Geometry: final body of the model. Coordinates: model frame, mm. A direction names the side the tool comes from. Coordinates: 2 decimals unless noted, no trailing zeros. Write each loop counter-clockwise with the first axis right and the second up, starting at its lowest first coordinate (ties: lowest second). Pieces come first, ordered by that corner, then holes. Notation, with made-up numbers: (49, 13) -> (97, 13) arc R17 cw to (97, 31) -> close; hole circle Ø10 at (8.25, 7.5). An arc over 180 degrees is marked (long way). Answer as a JSON object with one key per item and string values. Group by question number.
```python
from build123d import *

# Parameters (mm, degrees)
F1_DEPTH = 6
F3_DEPTH = 2
F4_R     = 2.25
F5_DEPTH = 8.001
F6_R     = 3.75
F7_DEPTH = 2
F8_SIZE  = 3


with BuildPart() as f1:
    # F0 (on Top) → F1 (new body)
    with BuildSketch(Plane.XY):
        Polygon((-30, 0), (-10, 0), (-10, -40), (0, -40), (10, -40), (10, 0), (30, 0), (30, 20), (0, 20), (-30, 20), align=None)
    extrude(amount=F1_DEPTH)

    # F2 (on face) → F3 (join)
    with BuildSketch(Plane.XY.offset(6)):
        Polygon((2.71, 0), (0, 0), (-2.71, 0), (-2.71, -40), (2.71, -40), align=None)
        Polygon((30, 7.29), (30, 12.71), (-30, 12.71), (-30, 10), (-30, 7.29), align=None)
    extrude(amount=F3_DEPTH)

    # F4 (on face) → F5 (cut, through all)
    with BuildSketch(Plane(origin=(0, 0, 0), x_dir=(1, 0, 0), z_dir=(0, 0, -1))):
        with Locations((-20, -10)):
            Circle(F4_R)
        with Locations((0, 10)):
            Circle(F4_R)
        with Locations((0, 30)):
            Circle(F4_R)
        with Locations((20.741304, -10)):
            Circle(F4_R)
        with Locations((0, -10)):
            Circle(F4_R)
    extrude(amount=-F5_DEPTH, mode=Mode.SUBTRACT)

    # F6 (on face) → F7 (cut)
    with BuildSketch(Plane(origin=(0, 0, 0), x_dir=(1, 0, 0), z_dir=(0, 0, -1))):
        with Locations((0, 30)):
            Circle(F6_R)
        with Locations((0, 10)):
            Circle(F6_R)
        with Locations((20.741304, -10)):
            Circle(F6_R)
        with Locations((-20, -10)):
            Circle(F6_R)
        with Locations((0, -10)):
            Circle(F6_R)
    extrude(amount=-F7_DEPTH, mode=Mode.SUBTRACT)

    # F8
    f8_edges = [f1.edges().sort_by_distance(p)[0] for p in [
        (-10, -20, 0),
        (-20, 0, 0),
        (10, -20, 0),
        (20, 0, 0),
        (0, 20, 0),
        (30, 10, 0),
        (-30, 10, 0),
        (0, -40, 0),
    ]]
    chamfer(f8_edges, length=F8_SIZE)


solid = f1.part
```
Item 1: Mould query, pull axis Y, two halves, no side actions, for faces 5 (the flat face through (2, -28, 2)), 6 (the flat face through (-30, 10, 5)), 7 (the flat face through (18, 1, 2)). Classes: +Y half, -Y half, draft (parallel to the pull), parting line (faces both ways), or undercut.
Item 2: Section A-A on z = 6.75. Output: boundary loops of the cut face in (x, y).
Item 3: Contact query for flat-ended pins moving along their axis: pin 1 (3.5 mm diameter, centred on x = 16.5, z = 4, fed in from -Y); pin 2 (8 mm diameter, centred on x = -21.5, y = 11, fed in from -Z); pin 3 (0.6 mm diameter, centred on y = -29.5, z = 6.5, fed in from -X); pin 4 (1.6 mm diameter, centred on x = -10.5, z = 7, fed in from -Y). Output: stop coordinate, or through.
Item 4: Set-up query: faces 1 (the cylindrical face through (-0.488, -13.718, 0.986)), 2 (the flat face through (9, -19, 2)), 3 (the flat face through (2.71, -20, 7)), 4 (the flat face through (20, 0, 4)). Return all of +Z, -Z, +X, -X, +Y, -Y with unobstructed straight access to the full face (end or side cutting, diameter ignored); none if empty.
Item 5: Section B-B on x = -20. Output: boundary loops of the cut face in (y, z), then the cut area to 3 significant figures.
Item 6: Section C-C on y = 10. Give the number of separate pieces and of enclosed holes in the cut face, then the cut area to 3 significant figures.
Item 7: Ray query, L1, parallel to X at y = 10, z = 5.75; L2, parallel to X at y = 11, z = 6; L3, parallel to Y at x = -20, z = 3.4. Return the intervals inside material, ascending. Write a range as [from, to].
Item 8: Section D-D on y = -30. Output: boundary loops of the cut face in (x, z).
Answer sheet:
{
 "1": {"face 5": "undercut", "face 6": "draft", "face 7": "-Y half"},
 "2": {"outline": "(-30, 7.29) -> (30, 7.29) -> (30, 12.71) -> (-30, 12.71) -> close; (-2.71, -40) -> (2.71, -40) -> (2.71, 0) -> (-2.71, 0) -> close; hole circle Ø4.5 at (-20, 10); hole circle Ø4.5 at (0, -30); hole circle Ø4.5 at (0, -10); hole circle Ø4.5 at (0, 10); hole circle Ø4.5 at (20.74, 10)"},
 "3": {"pin 1": "stops at y = 0", "pin 2": "stops at z = 0", "pin 3": "stops at x = -2.71", "pin 4": "stops at y = 7.29"},
 "4": {"face 1": "-Z", "face 2": "-Z, +X, -Y", "face 3": "+Z, +X, -Y", "face 4": "+Z, -Z, +X, -Y"},
 "5": {"outline": "(0, 3) -> (3, 0) -> (6.25, 0) -> (6.25, 2) -> (7.75, 2) -> (7.75, 8) -> (7.29, 8) -> (7.29, 6) -> (0, 6) -> close; (12.25, 2) -> (13.75, 2) -> (13.75, 0) -> (17, 0) -> (20, 3) -> (20, 6) -> (12.71, 6) -> (12.71, 8) -> (12.25, 8) -> close", "area": "79.8 mm^2"},
 "6": {"separate pieces": "4", "enclosed holes": "0", "area": "345 mm^2"},
 "7": {"L1": "x = [-30, -22.25], [-17.75, -2.25], [2.25, 18.49], [22.99, 30]", "L2": "x = [-30, -22.02], [-17.98, -2.02], [2.02, 18.73], [22.76, 30]", "L3": "y = [0, 7.75], [12.25, 20]"},
 "8": {"outline": "(-10, 3) -> (-7, 0) -> (-3.75, 0) -> (-3.75, 2) -> (-2.25, 2) -> (-2.25, 8) -> (-2.71, 8) -> (-2.71, 6) -> (-10, 6) -> close; (2.25, 2) -> (3.75, 2) -> (3.75, 0) -> (7, 0) -> (10, 3) -> (10, 6) -> (2.71, 6) -> (2.71, 8) -> (2.25, 8) -> close"}
}
